Model file for the job. Use its own axes, mm. A direction names the side the tool comes from. Round coordinates to 2 decimals unless told otherwise and drop trailing zeros. Order: outer loops, then holes, each group sorted by start corner. A loop starts at its lowest first (then second) coordinate and runs counter-clockwise, first axis right, second up. Notation, with made-up numbers: (14, 46.5) -> (46, 46.5) arc R24 cw to (46, 64.5) -> close; hole circle Ø4 at (59, 7.5). An arc over 180 degrees is marked (long way). Put each result on its own line as item: value. Start each with the question number.
Q1. 3-axis set-ups, long thin cutter, end or side, ignore diameter. For faces 1 (the face through (36, 2.5, 2)), 2 (the face through (-36, 2.5, 2)), 3 (the face through (2.5, -36, 2)): which of +Z, -Z, +X, -X, +Y, -Y reach the whole face in a straight line?
Q2. Pull direction Z, two halves, no side cores. Call faces 4 (the face through (30.701, 9.025, 2.465)), 5 (the face through (0, -30, 0)), 6 (the face through (27, 14.3, 2)), 7 (the face through (-27, 14.3, 2)): released by +Z, released by -Z, zero draft, split by the parting line, or undercut.
Q3. Cut at C-C, the plane y = -15. List the corners of the cut face in (x, z).
Q4. Probe L1, parallel to X at y = 0, z = 2.05; L2, parallel to Y at x = 0, z = 3.25; L3, parallel to X at y = -3.5, z = 4.15. List the from-to ranges inside material, lowest first.
Q5. Cut at B-B, the plane z = 2.4. List the corners of the cut face in (x, y).
Q6. Flat gauge pins, fed straight in: P1, Ø1.5, axis at x = -34.5, z = 2, coming from the -Y side; P2, Ø2, axis at x = 22.5, z = 2, coming from the +Y side; P3, Ø3, axis at y = -6.5, z = 4, coming from the +X side. Where does each tip first touch, or does it go through?
Q7. Cut at A-A, the plane y = 0. List the corners of the cut face in (x, z).
Q8. Cut at D-D, the plane x = 34. List the corners of the cut face in (y, z), and give its area (3 significant figures).
Autodesk Inventor part; units mm, degrees
ref_plane "YZ Plane" through (0, 0, 0) normal (1, 0, 0) x (0, 1, 0)
ref_plane "XZ Plane" through (0, 0, 0) normal (0, 1, 0) x (-1, 0, 0)
ref_plane "XY Plane" through (0, 0, 0) normal (0, 0, 1) x (1, 0, 0)
sketch "Sketch1" plane through (0, 0, 0) normal (0, 0, 1) x (1, 0, 0)
  arc A0 (-25.4018, 15) -> (25.4018, 15) centre (0, 0) ccw
  line L0 (-28.2666, 15) -> (-25.4018, 15)
  line L1 (25.4018, 15) -> (28.2666, 15)
  line L2 (-39, 2.5) -> (-32, 2.5)
  line L3 (-32, -2.5) -> (-39, -2.5)
  line L4 (-39, -2.5) -> (-39, 2.5)
  line L5 (-32, 2.5) -> (-31.9022, 2.5)
  line L6 (-32, -2.5) -> (-31.9022, -2.5)
  line L7 (2.5, -32) -> (2.5, -39)
  line L8 (2.5, -39) -> (-2.5, -39)
  line L9 (-2.5, -39) -> (-2.5, -32)
  line L10 (-2.5, -32) -> (-2.5, -31.9022)
  line L11 (2.5, -32) -> (2.5, -31.9022)
  line L12 (32, 2.5) -> (39, 2.5)
  line L13 (39, 2.5) -> (39, -2.5)
  line L14 (39, -2.5) -> (32, -2.5)
  line L15 (32, 2.5) -> (31.9022, 2.5)
  line L16 (32, -2.5) -> (31.9022, -2.5)
  arc A1 (-28.2666, 15) -> (-31.9022, 2.5) centre (0, 0) ccw
  arc A2 (-31.9022, -2.5) -> (-2.5, -31.9022) centre (0, 0) ccw
  arc A3 (2.5, -31.9022) -> (31.9022, -2.5) centre (0, 0) ccw
  arc A4 (31.9022, 2.5) -> (28.2666, 15) centre (0, 0) ccw
  dimension "d18" = 59
  dimension "d41" = 7
  dimension "d42" = 5
  dimension "d43" = 5
  dimension "d44" = 7
  dimension "d45" = 7
  dimension "d46" = 5
extrude "Extrusion2" add sketch "Sketch1" along normal blind 5
sketch "Sketch2" plane through (-28.2666, 15, 0) normal (0, 1, 0) x (1, 0, 0)
  line L0 (0.4325, -1.5) -> (2.4325, -1.5)
  line L1 (2.4325, -1.5) -> (2.4325, -3.5)
  line L2 (2.4325, -3.5) -> (0.4325, -3.5)
  line L3 (0.4325, -3.5) -> (0.4325, -1.5)
  point P0 (28.2666, 0)
  point P1 (1.4325, -2.5)
  dimension "d51" = 2
  dimension "d52" = 2
sketch "Sketch3" plane through (25.4018, 15, 0) normal (0, 1, 0) x (1, 0, 0)
  line L0 (0.4325, -1.5) -> (2.4325, -1.5)
  line L1 (2.4325, -1.5) -> (2.4325, -3.5)
  line L2 (2.4325, -3.5) -> (0.4325, -3.5)
  line L3 (0.4325, -3.5) -> (0.4325, -1.5)
  point P0 (-25.4018, 0)
  point P1 (1.4325, -2.5)
  dimension "d55" = 2
  dimension "d56" = 2
extrude "Extrusion3" cut sketch "Sketch2" against normal blind 0.7
extrude "Extrusion4" cut sketch "Sketch3" against normal blind 0.7
properties part number "Clip_TestFitV1"
Ans:
1. face 1: +Z, -Z, +X, +Y
1. face 2: +Z, -Z, -X, +Y
1. face 3: +Z, -Z, +X, -Y
2. face 4: zero draft
2. face 5: released by -Z
2. face 6: undercut
2. face 7: undercut
3. outline: (-28.27, 0) -> (-25.4, 0) -> (-25.4, 5) -> (-28.27, 5) -> close; (25.4, 0) -> (28.27, 0) -> (28.27, 5) -> (25.4, 5) -> close
4. L1: x = -39 to -29.5, 29.5 to 39
4. L2: y = -39 to -29.5
4. L3: x = -31.81 to -29.29, 29.29 to 31.81
5. outline: (-39, -2.5) -> (-31.9, -2.5) arc R32 ccw to (-2.5, -31.9) -> (-2.5, -39) -> (2.5, -39) -> (2.5, -31.9) arc R32 ccw to (31.9, -2.5) -> (39, -2.5) -> (39, 2.5) -> (31.9, 2.5) arc R32 ccw to (28.27, 15) -> (27.83, 15) -> (27.83, 14.3) -> (25.83, 14.3) -> (25.83, 15) -> (25.4, 15) arc R29.5 cw (long way) to (-25.4, 15) -> (-25.83, 15) -> (-25.83, 14.3) -> (-27.83, 14.3) -> (-27.83, 15) -> (-28.27, 15) arc R32 ccw to (-31.9, 2.5) -> (-39, 2.5) -> close
6. P1: stops at y = -2.5
6. P2: stops at y = -17.83
6. P3: stops at x = 31.61
7. outline: (-39, 0) -> (-29.5, 0) -> (-29.5, 5) -> (-39, 5) -> close; (29.5, 0) -> (39, 0) -> (39, 5) -> (29.5, 5) -> close
8. outline: (-2.5, 0) -> (2.5, 0) -> (2.5, 5) -> (-2.5, 5) -> close
8. area: 25.0 mm^2
